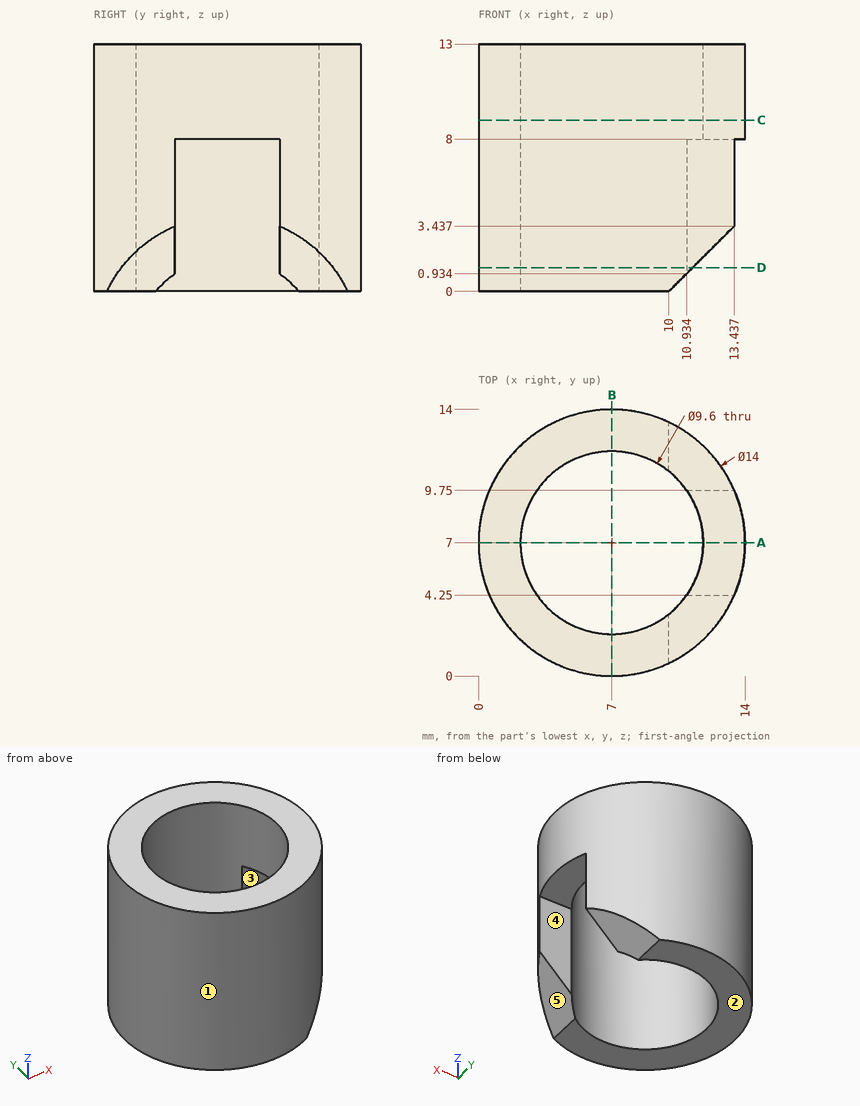
Here's the drawing with two shaded views (mm, measured from the low corner). I have some questions. A direction names the side the tool comes from. Round coordinates to 2 decimals unless told otherwise and drop trailing zeros. Order: outer loops, then holes, each group sorted by start corner. A loop starts at its lowest first (then second) coordinate and runs counter-clockwise, first axis right, second up. Notation, with made-up numbers: M 61,-12.75 L 78,-12.75 A15 ccw 78,-2.75 Z; hole C -37.75,-8.75 d11. An arc over 180 degrees is marked long. Use CSV: the item, a comma, the result in double quotes.
1) I want a section at D-D (z = 1.25). List the corners of the cut face in (x, y) for me.
Taken from the geometry:
outline,"M 10.93,4.25 A4.8 cw long 10.93,9.75 L 11.25,9.75 L 11.25,12.56 A7 ccw long 11.25,1.44 L 11.25,4.25 Z"
2) On a 3-axis mill with a long thin cutter (end or side, diameter ignored), from which of +Z, -Z, +X, -X, +Y, -Y can I reach the whole of each face in a straight line? I mean the marked faces 4 and 5. Say none if no direction works.
Taken from the geometry:
face 4,"-Z, +X"
face 5,"-Z, +X, +Y, -Y"
3) I want a section at A-A (y = 7). List the corners of the cut face in (x, z) for me, then the cut area to 3 significant figures.
Taken from the geometry:
outline,"M 0,0 L 2.2,0 L 2.2,13 L 0,13 Z; M 11.8,8 L 14,8 L 14,13 L 11.8,13 Z"
area,"39.6 mm^2"
4) I need wall thicknesses on line 1 along X through (y, z) = (7, 9); line 2 along Y through (x, z) = (6, 2.5) (1 decimal). Which ranges of each line are inside material? Lowest first, please. Write a range as [from, to].
Taken from the geometry:
line 1,"[0, 2.2], [11.8, 14]"
line 2,"[0.1, 2.3], [11.7, 13.9]"
5) I want a section at C-C (z = 9). List the corners of the cut face in (x, y) for me.
Taken from the geometry:
outline,"C 7,7 d14; hole C 7,7 d9.6"
6) I want a section at B-B (x = 7). List the corners of the cut face in (y, z) for me.
Taken from the geometry:
outline,"M 0,0 L 2.2,0 L 2.2,13 L 0,13 Z; M 11.8,0 L 14,0 L 14,13 L 11.8,13 Z"
7) I'm going to push flat-ended pins straight in: P1, Ø1.3, axis at x = 12, z = 4.5, coming from the -Y side; P2, Ø3.5, axis at x = 13, y = 6.5, coming from the -Z side; P3, Ø1.5, axis at x = 5, z = 11, coming from the +Y side. Where does each tip first touch, or does it pass through?
Taken from the geometry:
P1,"y = 1.52"
P2,"z = 8"
P3,"y = 13.89"
8) If we mould it in two halves opening along Y, with no side actions, what happens to the marked faces 1, 2 and 3? For each: pulls with the +Y half, pulls with the -Y half, needs draft (parallel to the pull), parting line crosses it, or undercut.
Taken from the geometry:
face 1,"parting line crosses it"
face 2,"needs draft"
face 3,"undercut"
